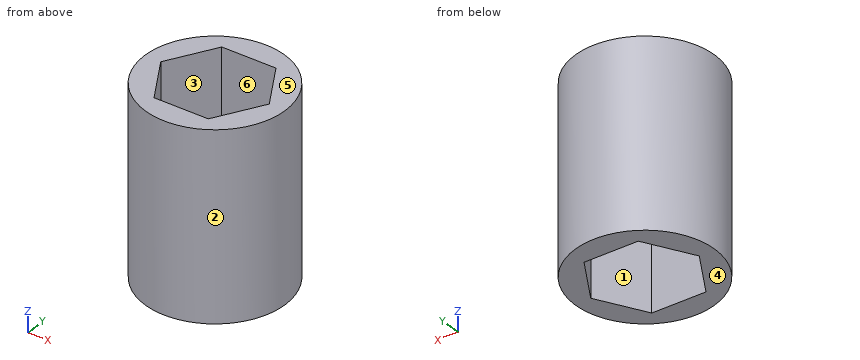
from build123d import *

# Parameters (mm, degrees)
SKETCH1_R           = 9.525
BOSS_EXTRUDE1_DEPTH = 25.2984


with BuildPart() as part:
    # Sketch1 → Boss-Extrude1 (new body)
    with BuildSketch(Plane.XY):
        Circle(SKETCH1_R)
        Polygon((-3.666174209, 6.35), (-7.332348419, 0), (-3.666174209, -6.35), (3.666174209, -6.35), (7.332348419, 0), (3.666174209, 6.35), align=None, mode=Mode.SUBTRACT)
    extrude(amount=BOSS_EXTRUDE1_DEPTH)


solid = part.part
Work out the finished part from the listing and answer in its coordinate system (mm). Face numbers are marked on the shaded views. A direction names the side the tool comes from. Round coordinates to 2 decimals unless told otherwise and drop trailing zeros. Loops run counter-clockwise (first coordinate to the right, second up) from the corner with the lowest first, then second, coordinate; pieces in that order, holes last. Notation, with made-up numbers: (47, 2) - (69, 2) arc R24 ccw to (69, 26) - close; hole circle Ø6 at (-16.75, -21). An arc over 180 degrees is marked (long way). One line per item, written item: value.
Q1. Each of these flat-tipped pins is pushed along its axis until it touches: pin 1 Ø2 at (x, z) = (-6.5, 21) entering from +Y; pin 2 Ø2 at (x, z) = (-7.5, 14) entering from +Y; pin 3 Ø8 at (y, z) = (7.5, 21) entering from -X. Where does it stop, or does it pass through?
Check values:
pin 1: y = 7.78
pin 2: y = 6.96
pin 3: x = -8.86
Q2. The mould has two halves that part along Y. Classify the marked faces 1, 2, 3 and 4: +Y half, -Y half, draft (parallel to the pull), parting line (faces both ways), or undercut.
Check values:
face 1: undercut
face 2: parting line
face 3: undercut
face 4: draft
Q3. Find section C-C on z = 23. Give the vertices of the cut face in (x, y) (3 decimals), and give its area (3 significant figures).
Check values:
outline: circle Ø19.05 at (0, 0); hole (-7.332, 0) - (-3.666, -6.35) - (3.666, -6.35) - (7.332, 0) - (3.666, 6.35) - (-3.666, 6.35) - close
area: 145 mm2
Q4. Find section D-D on y = -8. Give the vertices of the cut face in (x, z), and give its area (3 significant figures).
Check values:
outline: (-5.17, 0) - (5.17, 0) - (5.17, 25.3) - (-5.17, 25.3) - close
area: 262 mm2
Q5. For the marked faces 5 and 6, determine the directions among +Z, -Z, +X, -X, +Y, -Y from which every point of the face is accessible in a straight line to the end or side of a thin tool.
Check values:
face 5: +Z, +X, -X, +Y, -Y
face 6: +Z, -Z
Q6. Straight lines are drawn through the part: probe 1 along Y at (x, z) = (6.5, 20.25); probe 2 along X at (y, z) = (-6, 7.25); probe 3 along X at (y, z) = (-0.75, 20.5). For each, find the intervals that lie inside material, in ascending order.
Check values:
probe 1: -6.96 to -1.44, 1.44 to 6.96
probe 2: -7.4 to -3.87, 3.87 to 7.4
probe 3: -9.5 to -6.9, 6.9 to 9.5
Q7. Find section B-B on y = 2. Give the vertices of the cut face in (x, z), and give its area (3 significant figures).
Check values:
outline: (-9.31, 0) - (-6.18, 0) - (-6.18, 25.3) - (-9.31, 25.3) - close; (6.18, 0) - (9.31, 0) - (9.31, 25.3) - (6.18, 25.3) - close
area: 159 mm2
Q8. Find section A-A on x = 0. Give the vertices of the cut face in (y, z) (3 decimals).
Check values:
outline: (-9.525, 0) - (-6.35, 0) - (-6.35, 25.298) - (-9.525, 25.298) - close; (6.35, 0) - (9.525, 0) - (9.525, 25.298) - (6.35, 25.298) - close
